Autodesk Fusion 360 part; units mm, degrees
sketch "Sketch1" plane through (0, 0, 0) normal (0, 1, 0) x (1, 0, 0)
  circle A0 centre (0, 0) radius 3
  circle A1 centre (0, 0) radius 6.5
  circle A2 centre (0, 0) radius 7.5
  line L0 (-3.5081, -1.5) -> (3.6969, -1.5)
  line L1 (-2.4042, -1.7943) -> (-0.3233, -1.5)
  line L2 (-0.1362, -2.4721) -> (-1.3744, -2.6666)
  line L3 (-0.1362, -2.4721) -> (-0.2747, -1.4931)
  line L4 (-0.0006, -0.4974) -> (-0.0006, -3.2095)
  line L5 (-0.0006, -3.2095) -> (0.4355, -3.2095)
  line L6 (2.403, -1.7943) -> (0.3221, -1.5)
  line L7 (0.135, -2.4721) -> (0.2735, -1.4931)
  line L8 (0.135, -2.4721) -> (1.3732, -2.6666)
  line L9 (0.3221, -1.5) -> (0.2735, -1.4931)
  line L10 (-0.3233, -1.5) -> (-0.2747, -1.4931)
  line L11 (1.3732, -2.6666) -> (1.3779, -2.6674)
  line L12 (2.403, -1.7943) -> (2.4082, -1.7951)
  dimension "d1" = 6
  dimension "d2" = 13
  dimension "d3" = 15
  dimension "d4" = 1.5
  dimension "d5" = 0.4361
extrude "Extrude5" add sketch "Sketch1" along normal blind 1 contours A0 L0 L1 L2 L3 | A0 L0 L1 | A0 L0 L2 L3 L4 | A0 L0 L3 L7 L9 L10 | A0 L0 L4 L7 L8 | A0 L0 L6 L7 L8 | A0 L0 L6 | A1 | A2 makes body 1
extrude "Extrude2" add sketch "Sketch1" along normal blind 5 separate body contours A0 L0 L6 L7 L8 makes body 2
extrude "Extrude1" add sketch "Sketch1" along normal blind 5 separate body contours A0 L0 L1 L2 L3 makes body 3
extrude "Extrude3" add sketch "Sketch1" along normal blind 5 contours A1 bodies 2 3
extrude "Extrude4" add sketch "Sketch1" along normal blind -3 and the other way blind -5 separate body contours A2 makes body 4
move_body "Move1" bodies 1 to x (1, 0, 0) y (0, 1, 0) z (0, 0, 1) at (0, 5, 0)
combine "Combine1" operation add target body 4 tool bodies 1 2
chamfer "Chamfer1" distance 1.2 angle 45 1 edges at (-6.9925, 6, 2.7121) on bodies 4
Here's how the part is built. I have some questions about the finished solid (model axes, mm). A direction names the side the tool comes from. Coordinates: 2 decimals unless noted, no trailing zeros. Order: outer loops, then holes, each group sorted by start corner. A loop starts at its lowest first (then second) coordinate and runs counter-clockwise, first axis right, second up.
1) Imagine slicing it at B-B on y = 1. List the corners of the cut face in (x, z) for me (3 decimals), and give its area (3 significant figures).
2) We'd pull the mould along Z, two halves only. Please class faces 3 (the face through (0.2, 2.5, 2)), 4 (the face through (0, 6, 0)), 5 (the face through (-7.493, 0.955, -0.33)): +Z half, -Z half, draft (parallel to the pull), parting line (faces both ways), or undercut.
3) I need wall thicknesses on line 1 (X direction, y = -0.55, z = 0); line 2 (X direction, y = 2.4, z = 0). Which ranges of each line are inside material? Lowest first, please.
4) Imagine slicing it at C-C on y = -1.5. List the corners of the cut face in (x, z) for me, and give its area (3 significant figures).
5) Imagine slicing it at A-A on z = 0. List the corners of the cut face in (x, y) for me, and give its area (3 significant figures).
6) Which directions (+Z, -Z, +X, -X, +Y, -Y) give clear straight access to the entire face, cutting with the end or side of a thin tool? Please do faces 1 (the face through (-6, -3, -3)), 2 (the face through (-0.204, 2.465, 1.993)).
7) Will these pins go through, and if not, where does the flat tip stop? pin 1 (2 mm diameter, centred on x = 3, y = 3.5, fed in from -Z); pin 2 (5 mm diameter, centred on x = 0.5, z = 1, fed in from -Y).
Response values:
1. outline: circle Ø15 at (0, 0); hole (-2.404, 1.794) arc R3 ccw (long way) to (2.404, 1.795) - (0.322, 1.5) - (0.273, 1.5) - (0.135, 2.472) - (1.373, 2.667) arc R3 ccw to (-1.374, 2.667) - (-0.136, 2.472) - (-0.274, 1.5) - (-0.323, 1.5) - close
1. area: 152 mm2
2. face 3: undercut
2. face 4: draft
2. face 5: parting line
3. line 1: x = -7.5 to -6.5, 6.5 to 7.5
3. line 2: x = -7.5 to -3, 3 to 7.5
4. outline: circle Ø15 at (0, 0); hole circle Ø13 at (0, 0)
4. area: 44.0 mm2
5. outline: (-7.5, -3) - (-6.5, -3) - (-6.5, 0) - (-3, 0) - (-3, 5) - (3, 5) - (3, 0) - (6.5, 0) - (6.5, -3) - (7.5, -3) - (7.5, 4.8) - (6.3, 6) - (-6.3, 6) - (-7.5, 4.8) - close
5. area: 64.6 mm2
6. face 1: +Z, -Z, +X, -X, -Y
6. face 2: -Y
7. pin 1: stops at z = -7.23
7. pin 2: stops at y = 0
